Input: part model. Units: mm. Frame: model coordinates. Face numbers are marked on the shaded views. Round coordinates to 2 decimals unless told otherwise and drop trailing zeros. Loops run counter-clockwise (first coordinate to the right, second up) from the corner with the lowest first, then second, coordinate; pieces in that order, holes last.
(1) Draft query along Y for the marked faces 1, 2 and 3. Return one class per face: released by +Y, released by -Y, zero draft, split by the parting line, or undercut.
(2) Cut plane B-B, the plane x = 0. Output: boundary loops of the cut face in (y, z), and give its area (3 significant figures).
(3) Cut plane A-A, the plane x = 26. Output: boundary loops of the cut face in (y, z).
(4) Cut plane D-D, the plane y = -10. Output: boundary loops of the cut face in (x, z), and give its area (3 significant figures).
(5) Cut plane C-C, the plane z = 4.75. Output: boundary loops of the cut face in (x, y), and give its area (3 significant figures).
(6) Line query: line 1 (Y direction, x = 0, z = 2); line 2 (X direction, y = 24, z = 1.5) (3 decimals); line 3 (X direction, y = -7, z = 2.5). Output: solid intervals per line, ascending.
(7) First-contact query: pin 1 Ø19.5 at (x, y) = (-20.48, -11.82) entering from +Z; pin 2 Ø1.5 at (x, y) = (-10.5, 22) entering from +Z. Flat tips, straight axial feed; report the tip coordinate or a pass-through.
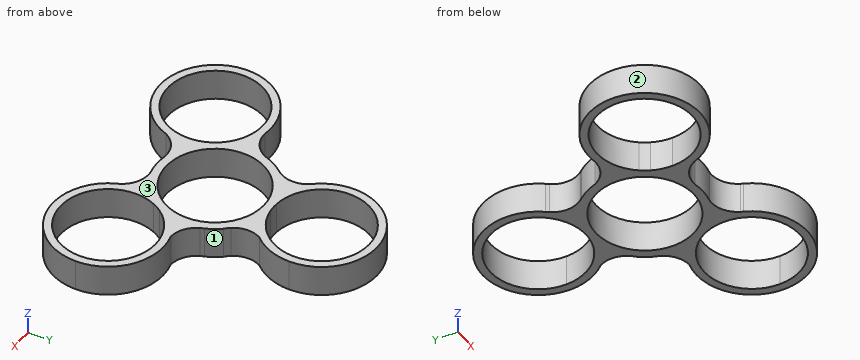
from build123d import *

# Parameters (mm, degrees)
F0_R     = 11.05
F1_DEPTH = 7


with BuildPart() as f1:
    # F0 (on Top) → F1 (new body)
    with BuildSketch(Plane.XY):
        with BuildLine():
            ThreePointArc((12.4036553845, 3.8922144215), (12.2588680886, 4.2668950825), (12.1397217876, 4.650500502))
            ThreePointArc((12.1397217876, 4.650500502), (11.3509584551, 6.3368558568), (10.3294036233, 7.8932515979))
            ThreePointArc((10.3294036233, 7.8932515979), (9.8245761866, 8.414561478), (9.3870501636, 8.9935137308))
            ThreePointArc((9.3870501636, 8.9935137308), (7.2468764963, 10.7927188904), (4.7714819389, 12.092682089))
            ThreePointArc((4.7714819389, 12.092682089), (0, 11.1461646855), (-4.7714819389, 12.092682089))
            ThreePointArc((-4.7714819389, 12.092682089), (-7.5081755961, 10.6126009639), (-9.8148092936, 8.5246418417))
            ThreePointArc((-9.8148092936, 8.5246418417), (-9.9218729104, 8.3943935706), (-10.0325882839, 8.2672348658))
            ThreePointArc((-10.0325882839, 8.2672348658), (-11.4424495934, 6.1701172844), (-12.419961597, 3.8398637906))
            ThreePointArc((-12.419961597, 3.8398637906), (-12.9624394617, 0.9875035204), (-12.8583108585, -1.9141164717))
            ThreePointArc((-12.8583108585, -1.9141164717), (-9.6528617724, -5.5730823427), (-8.0868289195, -10.1785656173))
            ThreePointArc((-8.0868289195, -10.1785656173), (-5.5850066858, -11.7391524532), (-2.7958525219, -12.695794921))
            ThreePointArc((-2.7958525219, -12.695794921), (0.0017952144, -12.999999876), (2.7993588265, -12.6950222592))
            ThreePointArc((2.7993588265, -12.6950222592), (5.5866277322, -11.7383810886), (8.0868289195, -10.1785656173))
            ThreePointArc((8.0868289195, -10.1785656173), (9.6528617724, -5.5730823427), (12.8583108585, -1.9141164717))
            ThreePointArc((12.8583108585, -1.9141164717), (12.9645293235, -0.9596767268), (13, 0))
            ThreePointArc((13, 0), (12.8500490271, 1.9688169038), (12.4036553845, 3.8922144215))
        make_face()
        Circle(F0_R, mode=Mode.SUBTRACT)
        with BuildLine():
            ThreePointArc((17.4129621968, 0.2952691949), (14.4052350934, 1.3931332806), (12.4036553845, 3.8922144215))
            ThreePointArc((12.4036553845, 3.8922144215), (12.8500490271, 1.9688169038), (13, 0))
            ThreePointArc((13, 0), (12.9645293235, -0.9596767268), (12.8583108585, -1.9141164717))
            ThreePointArc((12.8583108585, -1.9141164717), (15.0226216268, -0.5764432777), (17.4129621968, 0.2952691949))
        make_face()
        with BuildLine():
            ThreePointArc((4.7714819389, 12.092682089), (7.2468764963, 10.7927188904), (9.3870501636, 8.9935137308))
            ThreePointArc((9.3870501636, 8.9935137308), (8.402604273, 11.9865844679), (9.0866097244, 15.0622539383))
            ThreePointArc((9.0866097244, 15.0622539383), (7.0863435832, 13.3488963768), (4.7714819389, 12.092682089))
        make_face()
        with BuildLine():
            ThreePointArc((32.9781793197, -11.8230823427), (28.1572022381, -1.9598877782), (17.4129621968, 0.2952691949))
            ThreePointArc((17.4129621968, 0.2952691949), (15.0226216268, -0.5764432777), (12.8583108585, -1.9141164717))
            ThreePointArc((12.8583108585, -1.9141164717), (12.4453302152, -3.7568278952), (11.7697355483, -5.5202649505))
            ThreePointArc((11.7697355483, -5.5202649505), (23.7907862581, -1.5961993733), (31.2281793197, -11.8230823427))
            ThreePointArc((31.2281793197, -11.8230823427), (18.2335395964, -22.3361262651), (10.6655574569, -7.4327575054))
            ThreePointArc((10.6655574569, -7.4327575054), (9.4761735025, -8.8995581772), (8.0868289195, -10.1785656173))
            ThreePointArc((8.0868289195, -10.1785656173), (8.05547786, -13.2110623297), (8.7553384731, -16.161861259))
            ThreePointArc((8.7553384731, -16.161861259), (8.8665325035, -16.4239751001), (8.9650446915, -16.6911138785))
            ThreePointArc((8.9650446915, -16.6911138785), (22.9617067654, -24.0738819667), (32.9781793197, -11.8230823427))
        make_face()
        with BuildLine():
            ThreePointArc((-4.7714819389, 12.092682089), (0, 11.1461646855), (4.7714819389, 12.092682089))
            ThreePointArc((4.7714819389, 12.092682089), (2.9691567127, 12.6563860725), (1.1041780914, 12.9530224559))
            ThreePointArc((1.1041780914, 12.9530224559), (0, 12.8961646855), (-1.1041780914, 12.9530224559))
            ThreePointArc((-1.1041780914, 12.9530224559), (-2.9691567127, 12.6563860725), (-4.7714819389, 12.092682089))
        make_face()
        with BuildLine():
            ThreePointArc((1.1041780914, 12.9530224559), (2.9691567127, 12.6563860725), (4.7714819389, 12.092682089))
            ThreePointArc((4.7714819389, 12.092682089), (7.0863435832, 13.3488963768), (9.0866097244, 15.0622539383))
            ThreePointArc((9.0866097244, 15.0622539383), (11.6153480696, 19.027324006), (12.5, 23.6461646855))
            ThreePointArc((12.5, 23.6461646855), (-3.8986180344, 35.5226446952), (-10.0681243875, 16.2378672213))
            ThreePointArc((-10.0681243875, 16.2378672213), (-9.794102473, 15.9150690623), (-9.5437602938, 15.5735790121))
            ThreePointArc((-9.5437602938, 15.5735790121), (-7.3661863194, 13.5471895341), (-4.7714819389, 12.092682089))
            ThreePointArc((-4.7714819389, 12.092682089), (-2.9691567127, 12.6563860725), (-1.1041780914, 12.9530224559))
            ThreePointArc((-1.1041780914, 12.9530224559), (-7.2004369839, 31.6284079317), (10.75, 23.6461646855))
            ThreePointArc((10.75, 23.6461646855), (7.9822432462, 16.4457277016), (1.1041780914, 12.9530224559))
        make_face()
        with BuildLine():
            ThreePointArc((11.7697355483, -5.5202649505), (12.4453302152, -3.7568278952), (12.8583108585, -1.9141164717))
            ThreePointArc((12.8583108585, -1.9141164717), (9.6528617724, -5.5730823427), (8.0868289195, -10.1785656173))
            ThreePointArc((8.0868289195, -10.1785656173), (9.4761735025, -8.8995581772), (10.6655574569, -7.4327575054))
            ThreePointArc((10.6655574569, -7.4327575054), (11.168406229, -6.4480823427), (11.7697355483, -5.5202649505))
        make_face()
        with BuildLine():
            ThreePointArc((-9.8148092936, 8.5246418417), (-7.5081755961, 10.6126009639), (-4.7714819389, 12.092682089))
            ThreePointArc((-4.7714819389, 12.092682089), (-7.3661863194, 13.5471895341), (-9.5437602938, 15.5735790121))
            ThreePointArc((-9.5437602938, 15.5735790121), (-8.5203205537, 12.0045453967), (-9.8148092936, 8.5246418417))
        make_face()
        with BuildLine():
            ThreePointArc((8.7553384731, -16.161861259), (8.05547786, -13.2110623297), (8.0868289195, -10.1785656173))
            ThreePointArc((8.0868289195, -10.1785656173), (5.5866277322, -11.7383810886), (2.7993588265, -12.6950222592))
            ThreePointArc((2.7993588265, -12.6950222592), (6.3311702253, -13.4769842407), (8.7553384731, -16.161861259))
        make_face()
        with BuildLine():
            ThreePointArc((-8.6738467532, -15.9349836863), (-6.2358648809, -13.4062219399), (-2.7958525219, -12.695794921))
            ThreePointArc((-2.7958525219, -12.695794921), (-5.5850066858, -11.7391524532), (-8.0868289195, -10.1785656173))
            ThreePointArc((-8.0868289195, -10.1785656173), (-8.0053712958, -10.9990313741), (-7.9781793197, -11.8230823427))
            ThreePointArc((-7.9781793197, -11.8230823427), (-8.1533231931, -13.9082493527), (-8.6738467532, -15.9349836863))
        make_face()
        with BuildLine():
            ThreePointArc((-12.8583108585, -1.9141164717), (-12.9624394617, 0.9875035204), (-12.419961597, 3.8398637906))
            ThreePointArc((-12.419961597, 3.8398637906), (-14.8010494837, 1.2584054136), (-18.2237650289, 0.4719416997))
            ThreePointArc((-18.2237650289, 0.4719416997), (-15.3989388877, -0.4015536958), (-12.8583108585, -1.9141164717))
        make_face()
        with BuildLine():
            ThreePointArc((-7.9781793197, -11.8230823427), (-8.0053712958, -10.9990313741), (-8.0868289195, -10.1785656173))
            ThreePointArc((-8.0868289195, -10.1785656173), (-9.4761735025, -8.8995581772), (-10.6655574569, -7.4327575054))
            ThreePointArc((-10.6655574569, -7.4327575054), (-9.9651353974, -9.5784426194), (-9.7281793197, -11.8230823427))
            ThreePointArc((-9.7281793197, -11.8230823427), (-30.7050622892, -15.1356892812), (-11.7697355483, -5.5202649505))
            ThreePointArc((-11.7697355483, -5.5202649505), (-12.4453302152, -3.7568278952), (-12.8583108585, -1.9141164717))
            ThreePointArc((-12.8583108585, -1.9141164717), (-15.3989388877, -0.4015536958), (-18.2237650289, 0.4719416997))
            ThreePointArc((-18.2237650289, 0.4719416997), (-31.281368245, -18.1112544972), (-8.6738467532, -15.9349836863))
            ThreePointArc((-8.6738467532, -15.9349836863), (-8.1533231931, -13.9082493527), (-7.9781793197, -11.8230823427))
        make_face()
        with BuildLine():
            ThreePointArc((-10.6655574569, -7.4327575054), (-9.4761735025, -8.8995581772), (-8.0868289195, -10.1785656173))
            ThreePointArc((-8.0868289195, -10.1785656173), (-9.6528617724, -5.5730823427), (-12.8583108585, -1.9141164717))
            ThreePointArc((-12.8583108585, -1.9141164717), (-12.4453302152, -3.7568278952), (-11.7697355483, -5.5202649505))
            ThreePointArc((-11.7697355483, -5.5202649505), (-11.168406229, -6.4480823427), (-10.6655574569, -7.4327575054))
        make_face()
    extrude(amount=F1_DEPTH)


solid = f1.part
Reported:
1. face 1: undercut
1. face 2: split by the parting line
1. face 3: zero draft
2. outline: (-13, 0) - (-11.05, 0) - (-11.05, 7) - (-13, 7) - close; (11.05, 0) - (12.9, 0) - (12.9, 7) - (11.05, 7) - close; (34.4, 0) - (36.15, 0) - (36.15, 7) - (34.4, 7) - close
2. area: 38.8 mm2
3. outline: (-23.04, 0) - (-21.05, 0) - (-21.05, 7) - (-23.04, 7) - close; (-2.6, 0) - (-0.61, 0) - (-0.61, 7) - (-2.6, 7) - close
4. outline: (-32.84, 0) - (-31.07, 0) - (-31.07, 7) - (-32.84, 7) - close; (-9.88, 0) - (-4.7, 0) - (-4.7, 7) - (-9.88, 7) - close; (4.7, 0) - (9.88, 0) - (9.88, 7) - (4.7, 7) - close; (31.07, 0) - (32.84, 0) - (32.84, 7) - (31.07, 7) - close
4. area: 97.4 mm2
5. outline: (-18.22, 0.47) arc R12.5 ccw (long way) to (-8.67, -15.93) arc R5.94 cw to (-2.8, -12.7) arc R13 ccw to (2.8, -12.7) arc R5.94 cw to (8.97, -16.69) arc R12.5 ccw (long way) to (17.41, 0.3) arc R5.94 cw to (12.14, 4.65) arc R13 ccw to (10.33, 7.89) arc R5.94 cw to (9.09, 15.06) arc R12.5 ccw (long way) to (-10.07, 16.24) arc R5.94 cw to (-10.03, 8.27) arc R13 ccw to (-12.42, 3.84) arc R5.94 cw to start; hole circle Ø21.5 at (-20.48, -11.82); hole circle Ø22.1 at (0, 0); hole circle Ø21.5 at (0, 23.65); hole circle Ø21.5 at (20.48, -11.82)
5. area: 546 mm2
6. line 1: y = -13 to -11.05, 11.05 to 12.9, 34.4 to 36.15
6. line 2: x = -12.495 to -10.744, 10.744 to 12.495
6. line 3: x = -32.01 to -30.09, -10.87 to -8.55, 8.55 to 10.87, 30.09 to 32.01
7. pin 1: passes through
7. pin 2: stops at z = 7
